from build123d import *

# Parameters (mm, degrees)
SKETCH1_W           = 17
SKETCH1_H           = 28
BOSS_EXTRUDE1_DEPTH = 0.8
SKETCH3_W           = 8.4
SKETCH3_H           = 8
BOSS_EXTRUDE2_DEPTH = 2.7
CUT_EXTRUDE1_DEPTH  = 7.7


with BuildPart() as part:
    # Sketch1 → Boss-Extrude1 (new body)
    with BuildSketch(Plane(origin=(0, 0, 0), x_dir=(1, 0, 0), z_dir=(0, 1, 0))):
        Rectangle(SKETCH1_W, SKETCH1_H)
    extrude(amount=BOSS_EXTRUDE1_DEPTH)

    # Sketch3 → Boss-Extrude2 (add)
    with BuildSketch(Plane(origin=(0, 0.8, 0), x_dir=(1, 0, 0), z_dir=(0, 1, 0))):
        with Locations((0, 11.5)):
            Rectangle(SKETCH3_W, SKETCH3_H)
    extrude(amount=BOSS_EXTRUDE2_DEPTH)

    # Sketch4 → Cut-Extrude1 (cut)
    with BuildSketch(Plane(origin=(0, 0, -15.5), x_dir=(-1, 0, 0), z_dir=(0, 0, -1))):
        with BuildLine():
            ThreePointArc((-4.2, 2.15), (-3.804594155, 3.104594155), (-2.85, 3.5))
            Line((-2.85, 3.5), (-4.2, 3.5))
            Line((-4.2, 3.5), (-4.2, 2.15))
        make_face()
        with BuildLine():
            ThreePointArc((-2.85, 0.8), (-3.804594155, 1.195405845), (-4.2, 2.15))
            Line((-4.2, 2.15), (-4.2, 0.8))
            Line((-4.2, 0.8), (-2.85, 0.8))
        make_face()
        with BuildLine():
            Line((4.2, 0.8), (4.2, 2.15))
            ThreePointArc((4.2, 2.15), (3.804594155, 1.195405845), (2.85, 0.8))
            Line((2.85, 0.8), (4.2, 0.8))
        make_face()
        with BuildLine():
            Line((4.2, 3.5), (2.85, 3.5))
            ThreePointArc((2.85, 3.5), (3.804594155, 3.104594155), (4.2, 2.15))
            Line((4.2, 2.15), (4.2, 3.5))
        make_face()
        with BuildLine():
            Line((-2.85, 1.05), (2.85, 1.05))
            ThreePointArc((2.85, 1.05), (3.95, 2.15), (2.85, 3.25))
            Line((2.85, 3.25), (-2.85, 3.25))
            ThreePointArc((-2.85, 3.25), (-3.95, 2.15), (-2.85, 1.05))
        make_face()
        with BuildLine():
            ThreePointArc((2.85, 1.8), (3.2, 2.15), (2.85, 2.5))
            Line((2.85, 2.5), (-2.85, 2.5))
            ThreePointArc((-2.85, 2.5), (-3.2, 2.15), (-2.85, 1.8))
            Line((-2.85, 1.8), (2.85, 1.8))
        make_face(mode=Mode.SUBTRACT)
    extrude(amount=-CUT_EXTRUDE1_DEPTH, mode=Mode.SUBTRACT)


solid = part.part
Verification items for the finished model (mm, model axes). A direction names the side the tool comes from. Coordinates: 2 decimals unless noted, no trailing zeros. Order: outer loops, then holes, each group sorted by start corner. A loop starts at its lowest first (then second) coordinate and runs counter-clockwise, first axis right, second up. Notation, with made-up numbers: (-23.75, 29.5) -> (35.25, 29.5) arc R16 cw to (35.25, 38.5) -> close; hole circle Ø3 at (-36.75, 22). An arc over 180 degrees is marked (long way). Put each result on its own line as item: value. Start each with the question number.
1. Cross-section at A-A, the plane x = -1. Record the boundary of the cut face in (y, z).
2. Cross-section at C-C, the plane z = -1.75. Record the boundary of the cut face in (x, y), then the cut area to 3 significant figures.
3. Go/stop test with flat-tipped pins: pin 1 Ø1 at (x, y) = (-6, 2) entering from -Z; pin 2 Ø8 at (x, z) = (-5, -2.5) entering from +Y; pin 3 Ø1.5 at (y, z) = (1.5, 9) entering from +X; pin 4 Ø2 at (x, y) = (-1, 2.5) entering from +Z. Record where each tip stops, or that it passes through.
4. Cross-section at B-B, the plane y = 0.45. Record the boundary of the cut face in (x, z).
5. Material ranges on L1, parallel to Y at x = -0.25, z = -8; L2, parallel to Y at x = 3.5, z = -3; L3, parallel to Z at x = 1.5, y = 2.75, recorded low to high. Write a range as [from, to].
6. Cross-section at D-D, the plane x = -3.5. Record the boundary of the cut face in (y, z), then the cut area to 3 significant figures.
7. Access from +Z, -Z, +X, -X, +Y, -Y to the whole of each face (thin tool, end or side, straight path). Record for faces 4 (the flat face through (4, 3.2, -7.8)), 5 (the flat face through (0, 2, -7.5)), 6 (the flat face through (0, 1.05, -12)), 7 (the flat face through (4, 1, -7.8)).
8. Mould release check, pull along Y, two halves, no side actions. Record for faces 1 (the flat face through (-3.9, 3.3, -7.8)), 2 (the cylindrical face through (-3.95, 2.13, -11.7)), 3 (the flat face through (0, 0.8, -15)): released by +Y, released by -Y, zero draft, split by the parting line, or undercut.
Computed:
1. outline: (0, -14) -> (0.8, -14) -> (0.8, -15.5) -> (1.05, -15.5) -> (1.05, -7.8) -> (1.8, -7.8) -> (1.8, -15.5) -> (2.5, -15.5) -> (2.5, -7.8) -> (3.25, -7.8) -> (3.25, -15.5) -> (3.5, -15.5) -> (3.5, -7.5) -> (0.8, -7.5) -> (0.8, 14) -> (0, 14) -> close
2. outline: (-8.5, 0) -> (8.5, 0) -> (8.5, 0.8) -> (-8.5, 0.8) -> close
2. area: 13.6 mm2
3. pin 1: through
3. pin 2: y = 0.8
3. pin 3: x = 8.5
3. pin 4: z = -7.5
4. outline: (-8.5, -14) -> (8.5, -14) -> (8.5, 14) -> (-8.5, 14) -> close
5. L1: [0, 1.05], [1.8, 2.5], [3.25, 3.5]
5. L2: [0, 0.8]
5. L3: [-7.8, -7.5]
6. outline: (0, -14) -> (0.8, -14) -> (0.8, -7.8) -> (0.97, -7.8) -> (0.97, -15.5) -> (1.26, -15.5) -> (1.26, -7.8) -> (3.04, -7.8) -> (3.04, -15.5) -> (3.33, -15.5) -> (3.33, -7.8) -> (3.5, -7.8) -> (3.5, -7.5) -> (0.8, -7.5) -> (0.8, 14) -> (0, 14) -> close
6. area: 27.8 mm2
7. face 4: -Z, +X, +Y
7. face 5: +Z, +X, -X, +Y
7. face 6: -Z
7. face 7: -Z, +X
8. face 1: zero draft
8. face 2: undercut
8. face 3: released by -Y
